Autodesk Inventor part; units mm, degrees
ref_plane "YZ Plane" through (0, 0, 0) normal (1, 0, 0) x (0, 1, 0)
ref_plane "XZ Plane" through (0, 0, 0) normal (0, 1, 0) x (-1, 0, 0)
ref_plane "XY Plane" through (0, 0, 0) normal (0, 0, 1) x (1, 0, 0)
sketch "Sketch1" plane through (0, 0, 0) normal (0, 0, 1) x (1, 0, 0)
  line L0 (81.4908, -72.5941) -> (81.4908, 27.3941)
  line L1 (79.0849, 29.8) -> (81.4908, 27.3941)
  line L2 (-20.9033, 29.8) -> (79.0849, 29.8)
  line L3 (-23.3092, 27.3941) -> (-20.9033, 29.8)
  line L4 (-23.3092, -72.5941) -> (-23.3092, 27.3941)
  line L5 (-20.9033, -75) -> (-23.3092, -72.5941)
  line L6 (-4.3092, -75) -> (-20.9033, -75)
  line L7 (-4.3092, -73) -> (-4.3092, -75)
  line L8 (-4.3092, -73) -> (-20.0749, -73)
  line L9 (-21.3092, -71.7657) -> (-21.3092, 26.5657)
  line L10 (78.2565, 27.8) -> (-20.0749, 27.8)
  line L11 (79.4908, 26.5657) -> (78.2565, 27.8)
  line L12 (79.4908, -71.7657) -> (79.4908, 26.5657)
  line L13 (79.4908, -71.7657) -> (78.2565, -73)
  line L14 (78.2565, -73) -> (32.1708, -73)
  line L15 (32.1708, -75) -> (32.1708, -73)
  line L16 (79.0849, -75) -> (32.1708, -75)
  line L17 (79.0849, -75) -> (81.4908, -72.5941)
  line L18 (-4.3092, -75) -> (-23.3092, -75)
  line L19 (-23.3092, -75) -> (-23.3092, -73)
  line L20 (-23.3092, -73) -> (-4.3092, -73)
  line L21 (-4.3092, -73) -> (-4.3092, -75)
  line L22 (-21.3092, -59.0157) -> (-23.3092, -59.0157)
  line L23 (-23.3092, -59.0157) -> (-23.3092, -75)
  line L24 (-23.3092, -75) -> (-21.3092, -75)
  line L25 (-21.3092, -75) -> (-21.3092, -59.0157)
  line L26 (-20.9092, 18.65) -> (-20.9092, 26.4) construction
  line L27 (-20.9092, 26.4) -> (-19.9092, 27.4) construction
  line L28 (-19.9092, 27.4) -> (-12.1888, 27.4) construction
  line L29 (-21.3092, 18.65) -> (-21.3092, 26.5657)
  line L30 (-21.3092, 26.5657) -> (-20.0749, 27.8)
  line L31 (-20.0749, 27.8) -> (-12.1888, 27.8)
  line L32 (-22.7184, -70.3564) -> (-18.2476, -74.8272)
  line L33 (-22.7184, -70.3564) -> (-16.3958, -70.3564) construction
  line L34 (-4.3092, -75) -> (32.1708, -75)
  line L35 (32.1708, -75) -> (32.1708, -47)
  line L36 (32.1708, -47) -> (-4.3092, -47)
  line L37 (-4.3092, -47) -> (-4.3092, -75)
  circle A0 centre (-17.5342, -45.35) radius 1.75
  circle A1 centre (73.986, 22.4207) radius 1.75
  circle A2 centre (75.015, -68.5242) radius 1.75
  line L38 (-20.0749, -73) -> (-21.3092, -71.7657)
  line L39 (-21.3092, 26.5657) -> (-20.0749, 27.8)
  point P0 (0, 0)
  point P1 (-7.3249, -73)
  point P2 (-21.3092, -71.7657)
  point P3 (-20.0749, -73)
  point P4 (-17.9077, 27.8)
  point P5 (-21.3092, 18.65)
  point P6 (-21.3092, -74.5941)
extrude "Extrusion1" add sketch "Sketch1" against normal blind 3 contours L35 L36 L37 L8 L32 L9 L30 L10 L11 L12 L13 L14
sketch "Sketch2" plane through (0, 0, 0) normal (0, 0, 1) x (1, 0, 0)
  line L0 (-21.3092, -71.7657) -> (-21.3092, 26.5657)
  line L1 (-21.3092, 5.65) -> (-13.8092, 5.65)
  line L2 (-13.8092, 5.65) -> (-13.8092, -41.85)
  line L3 (-13.8092, -41.85) -> (-21.3092, -41.85)
  line L4 (-21.3092, -41.85) -> (-21.3092, 5.65)
  circle A0 centre (-17.5342, -45.35) radius 1.75
  point P0 (0, 0)
  point P1 (-17.5592, 5.65)
  dimension "d6" = 7.5
  dimension "d7" = 3.5
  dimension "d8" = 47.5
extrude "Extrusion2" cut sketch "Sketch2" against normal blind 3 contours L0 L1 L2 L3
sketch "Sketch3" plane through (0, 0, 0) normal (0, 0, 1) x (1, 0, 0)
  circle A0 centre (-17.5342, -45.35) radius 1.75
  point P0 (0, 0)
extrude "Extrusion3" add sketch "Sketch3" against normal up to surface (3 mm away)
sketch "Sketch4" plane through (0, 0, 0) normal (0, 0, 1) x (1, 0, 0)
  line L0 (-3.3235, -61.1555) -> (-1.2915, -61.1555)
  line L1 (0.4425, -54.1555) -> (-5.0575, -54.1555)
  line L2 (-5.0575, -54.1555) -> (-5.0575, -68.1555)
  line L3 (-5.0575, -68.1555) -> (0.4425, -68.1555)
  line L4 (0.4425, -68.1555) -> (0.4425, -54.1555)
  line L5 (0.4425, -54.1555) -> (-5.0575, -68.1555) construction
  line L6 (-5.0575, -54.1555) -> (0.4425, -68.1555) construction
  point P0 (0, 0)
  point P1 (-2.3075, -61.1555)
  dimension "d13" = 5.5
  dimension "d14" = 14
extrude "Extrusion4" cut sketch "Sketch4" against normal up to surface (3 mm away)
sketch "Sketch5" plane through (0, 0, 0) normal (0, 0, 1) x (1, 0, 0)
  point P0 (0, 0)
sketch "Sketch6" plane through (0, 0, 0) normal (0, 0, 1) x (1, 0, 0)
  line L0 (-5.0575, -54.1555) -> (-4.3092, -54.1555)
  line L1 (-4.3092, -54.1555) -> (-4.3092, -47)
  line L2 (-4.3092, -47) -> (32.1708, -47)
  line L3 (32.1708, -47) -> (32.1708, -73)
  line L4 (32.1708, -73) -> (78.2565, -73)
  line L5 (78.2565, -73) -> (79.4908, -71.7657)
  line L6 (79.4908, -71.7657) -> (79.4908, 26.5657)
  line L7 (79.4908, 26.5657) -> (78.2565, 27.8)
  line L8 (78.2565, 27.8) -> (-20.0749, 27.8)
  line L9 (-20.0749, 27.8) -> (-21.3092, 26.5657)
  line L10 (-21.3092, 26.5657) -> (-21.3092, 5.65)
  line L11 (-21.3092, 5.65) -> (-13.8092, 5.65)
  line L12 (-13.8092, 5.65) -> (-13.8092, -41.85)
  line L13 (-13.8092, -41.85) -> (-21.3092, -41.85)
  line L14 (-21.3092, -41.85) -> (-21.3092, -71.7657)
  line L15 (-21.3092, -71.7657) -> (-20.0749, -73)
  line L16 (-20.0749, -73) -> (-4.3092, -73)
  line L17 (-4.3092, -73) -> (-4.3092, -68.1555)
  line L18 (-4.3092, -68.1555) -> (-5.0575, -68.1555)
  line L19 (-5.0575, -68.1555) -> (-5.0575, -54.1555)
  circle A0 centre (75.015, -68.5242) radius 1.75
  circle A1 centre (73.986, 22.4207) radius 1.75
  line L20 (32.1708, -73) -> (38.1708, -73)
  line L21 (38.1708, -73) -> (38.1708, -47)
  line L22 (38.1708, -47) -> (32.1708, -47)
  line L23 (32.1708, -47) -> (32.1708, -73)
  point P0 (0, 0)
  dimension "d17" = 6
extrude "Extrusion5" cut sketch "Sketch6" against normal blind 10 contours L22 L21 L4 L3
properties part number "Lid_clear"
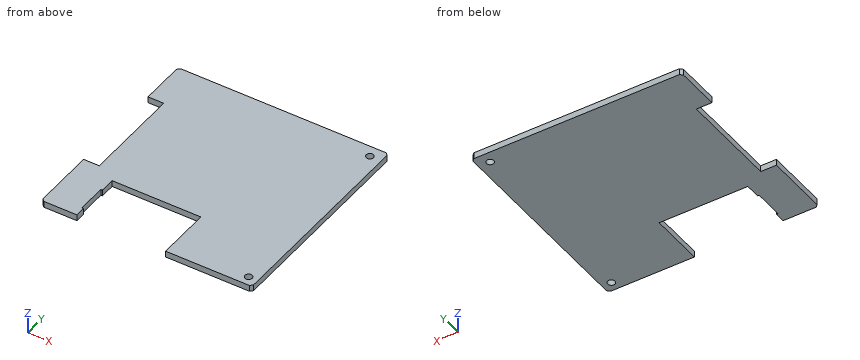
Could you check a few things on this model? Use its own coordinates, in mm. Give positions to 0.01 mm unless a question says otherwise; leave off trailing zeros. Loops run counter-clockwise (first coordinate to the right, second up) from the corner with the lowest first, then second, coordinate; pieces in that order, holes last. Notation, with made-up numbers: M 55,89 L 70,89 A34 ccw 70,124 Z; hole C 39,76 d10. An arc over 180 degrees is marked long. Answer as a JSON object with one key per item and string values.
Q1. Suppose I cut it at A-A, the plane z = -0.95. State how many separate pieces and enclosed holes the cut face has, plus the area to 3 significant figures.
Values found:
{"separate pieces": "1", "enclosed holes": "2", "area": "8,670 mm²"}
Q2. Suppose I cut it at B-B, the plane y = -14. List the corners of the cut face in (x, z) for me.
Values found:
{"outline": "M -13.81,-3 L 79.49,-3 L 79.49,0 L -13.81,0 Z"}
Q3. Suppose I cut it at C-C, the plane x = 34. List the corners of the cut face in (y, z) for me, plus the area to 3 significant figures.
Values found:
{"outline": "M -47,-3 L 27.8,-3 L 27.8,0 L -47,0 Z", "area": "224 mm²"}
Q4. If I drill on probe 1 along Y at (x, z) = (73.5, -1.5); probe 2 along X at (y, z) = (-68, -1.1); probe 3 along X at (y, z) = (-57, -0.8), over which ranges is the centre line in solid material (lowest first)? Write a range as [from, to].
Values found:
{"probe 1": "y = [-73, -69.4], [-67.65, 20.74], [24.1, 27.8]", "probe 2": "x = [-21.31, -5.06], [38.17, 73.35], [76.68, 79.49]", "probe 3": "x = [-21.31, -5.06], [38.17, 79.49]"}
